Could you check a few things on this drawing? It's one solid part, dimensions in mm from its lowest x, y, z. A direction names the side the tool comes from. Coordinates: 2 decimals unless noted, no trailing zeros. Loops run counter-clockwise (first coordinate to the right, second up) from the corner with the lowest first, then second, coordinate; pieces in that order, holes last. Notation, with made-up numbers: (77.25, 40) -> (117.25, 40) arc R23 cw to (117.25, 72) -> close; hole circle Ø1 at (76.25, 56.5). An arc over 180 degrees is marked (long way). One line per question, with ' | ' between items.
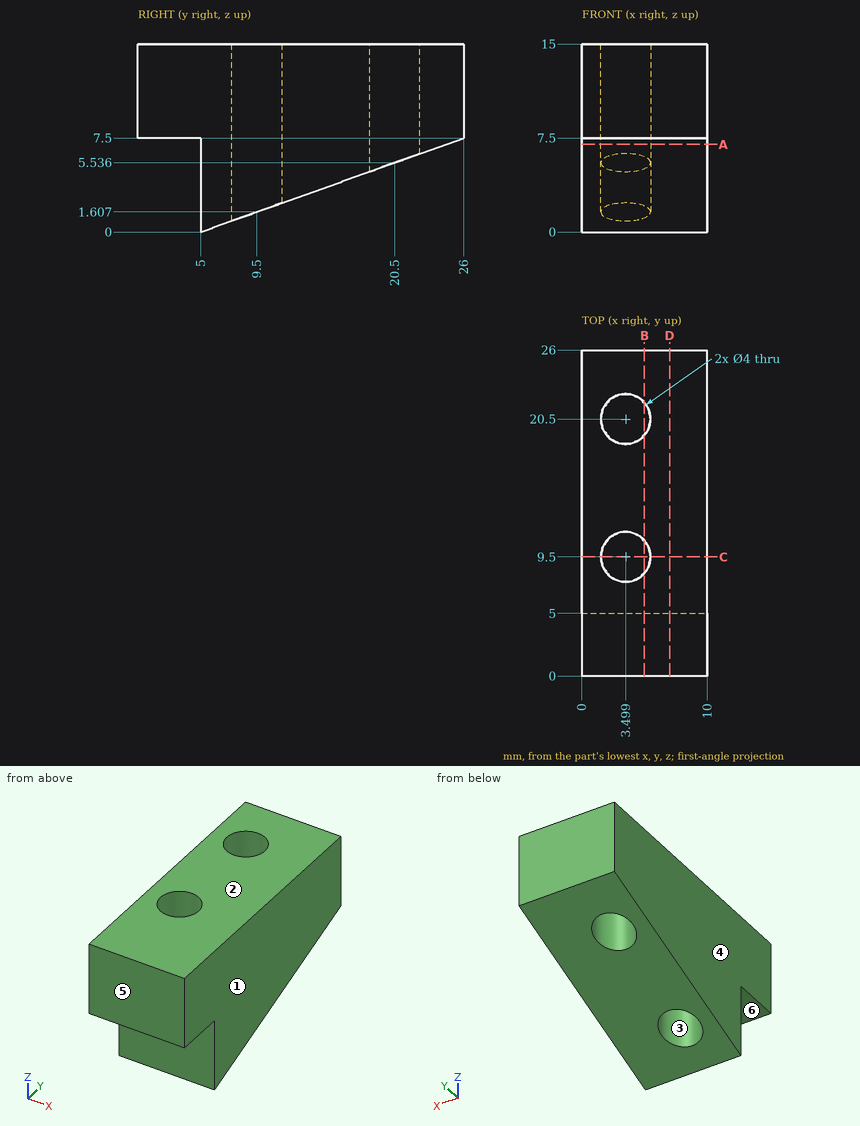
1) If we section it at B-B on x = 5: Please give me the cut outline in (y, z) (1 decimal), and give its area (3 significant figures).
Data:
outline: (0, 7.5) -> (5, 7.5) -> (5, 0) -> (8.2, 1.1) -> (8.2, 15) -> (0, 15) -> close; (10.8, 2.1) -> (19.2, 5.1) -> (19.2, 15) -> (10.8, 15) -> close; (21.8, 6) -> (26, 7.5) -> (26, 15) -> (21.8, 15) -> close | area: 213 mm²
2) I need wall thicknesses on line 1 along X through (y, z) = (9.5, 9.5); line 2 along Y through (x, z) = (3.5, 1); line 3 along Z through (x, y) = (6, 4.5). Which ranges of each line are inside material? Lowest first, please. Write a range as from..to.
Data:
line 1: 0..1.5, 5.5..10 | line 2: 5..7.5 | line 3: 7.5..15
3) If we section it at A-A on z = 7: Please give me the cut outline in (x, y), and give its area (3 significant figures).
Data:
outline: (0, 5) -> (10, 5) -> (10, 24.6) -> (0, 24.6) -> close; hole circle Ø4 at (3.5, 9.5); hole circle Ø4 at (3.5, 20.5) | area: 171 mm²
4) On a 3-axis mill with a long thin cutter (end or side, diameter ignored), from which of +Z, -Z, +X, -X, +Y, -Y can I reach the whole of each face in a straight line? I mean the marked faces 5 and 6. Say none if no direction works.
Data:
face 5: +Z, -Z, +X, -X, -Y | face 6: -Z, +X, -X, -Y
5) If we section it at D-D on x = 7: Please give me the cut outline in (y, z), and give its area (3 significant figures).
Data:
outline: (0, 7.5) -> (5, 7.5) -> (5, 0) -> (26, 7.5) -> (26, 15) -> (0, 15) -> close | area: 274 mm²
6) If we section it at C-C on y = 9.5: Please give me the cut outline in (x, z).
Data:
outline: (0, 1.61) -> (1.5, 1.61) -> (1.5, 15) -> (0, 15) -> close; (5.5, 1.61) -> (10, 1.61) -> (10, 15) -> (5.5, 15) -> close
7) We'd pull the mould along X, two halves only. Please class the marked faces 1, 2, 3 and 4: pulls with the +X half, pulls with the -X half, needs draft (parallel to the pull), parting line crosses it, or undercut.
Data:
face 1: pulls with the +X half | face 2: needs draft | face 3: undercut | face 4: pulls with the -X half
8) I'm going to push flat-ended pins straight in: pin 1 Ø4 at (x, z) = (2, 12.5) entering from -Y; pin 2 Ø1.5 at (x, y) = (6, 12.5) entering from -Z; pin 3 Ø5.5 at (x, y) = (2.5, 1.5) entering from -Z. Where does each tip first touch, or does it pass through?
Data:
pin 1: y = 0 | pin 2: z = 2.41 | pin 3: z = 7.5
